```python
from build123d import *

# Parameters (mm, degrees)
F1_DEPTH = 22.86
F3_DEPTH = 1.2192


with BuildPart() as f1:
    # F0 (on Front) → F1 (new body)
    with BuildSketch(Plane.XZ):
        Polygon((0, 1.2192), (0, 0), (19.812, 0), (19.812, 1.2192), (18.5928, 1.2192), (18.5928, 2.4384), (1.2192, 2.4384), (1.2192, 1.2192), align=None)
    extrude(amount=F1_DEPTH)

    # F2 (on face) → F3 (join)
    with BuildSketch(Plane.XZ.offset(22.86)):
        Polygon((0, 1.2192), (0, 0), (19.812, 0), (19.812, 1.2192), (18.5928, 1.2192), (1.2192, 1.2192), align=None)
    extrude(amount=F3_DEPTH)


solid = f1.part
```
Work out the finished part from the listing and answer in its coordinate system (mm). A direction names the side the tool comes from. Give positions to 0.01 mm unless a question says otherwise; leave off trailing zeros. Loops run counter-clockwise (first coordinate to the right, second up) from the corner with the lowest first, then second, coordinate; pieces in that order, holes last. Notation, with made-up numbers: (59, -2.5) -> (74, -2.5) arc R11 cw to (74, 16.5) -> close; hole circle Ø7 at (-23.75, 62). An arc over 180 degrees is marked (long way). Put each result on its own line as item: value. Start each with the question number.
Item 1: The part is cut by section C-C (z = 2.05). Give the vertices of the cut face in (x, y).
Item 2: The part is cut by section B-B (x = 10). Give the vertices of the cut face in (y, z).
Item 3: Find the intervals of material crossed by L1, parallel to Y at x = 4.75, z = 2; L2, parallel to X at y = -6.5, z = 2; L3, parallel to Z at x = 1, y = -17.25, in increasing order. Write a range as [from, to].
Item 4: This flat-tipped pin is pushed along its axis until it touches: P1, Ø1.3, axis at y = -8.5, z = 2, coming from the +X side. Where does it stop, or does it pass through?
Item 5: Which of the six approach directions +Z, -Z, +X, -X, +Y, -Y give full straight-line access (tool end or side, diameter ignored) to faces 1 (the face through (18.593, -11, 2)), 2 (the face through (10, -22.86, 2)), 3 (the face through (1.219, -11, 2))?
Item 6: The part is cut by section A-A (y = -11.5). Give the vertices of the cut face in (x, z).
Answers below:
1. outline: (1.22, -22.86) -> (18.59, -22.86) -> (18.59, 0) -> (1.22, 0) -> close
2. outline: (-24.08, 0) -> (0, 0) -> (0, 2.44) -> (-22.86, 2.44) -> (-22.86, 1.22) -> (-24.08, 1.22) -> close
3. L1: [-22.86, 0]
3. L2: [1.22, 18.59]
3. L3: [0, 1.22]
4. P1: x = 18.59
5. face 1: +Z, +X, +Y, -Y
5. face 2: +Z, +X, -X, -Y
5. face 3: +Z, -X, +Y, -Y
6. outline: (0, 0) -> (19.81, 0) -> (19.81, 1.22) -> (18.59, 1.22) -> (18.59, 2.44) -> (1.22, 2.44) -> (1.22, 1.22) -> (0, 1.22) -> close
